```python
from build123d import *

# Parameters (mm, degrees)
F0_W     = 100
F0_H     = 40
F1_DEPTH = 3
F2_R     = 3
F3_W     = 18
F3_H     = 9
F4_DEPTH = 25
F5_R     = 4.49999
F6_R     = 4.49999


# Not quite as in the source:
# - a fillet or chamfer is up to 0.001 mm smaller than in the source, because OpenCascade refuses the exact size


with BuildPart() as f1:
    # F0 (on Top) → F1 (new body)
    with BuildSketch(Plane.XY):
        Rectangle(F0_W, F0_H)
    extrude(amount=F1_DEPTH)

    # F2
    f2_edges = [f1.edges().sort_by_distance(p)[0] for p in [
        (50, -20, 1.5),
        (50, 20, 1.5),
        (-50, -20, 1.5),
        (-50, 20, 1.5),
    ]]
    fillet(f2_edges, radius=F2_R)

    # F3 (on face) → F4 (cut)
    with BuildSketch(Plane.XY.offset(3)):
        with Locations((-35, 0)):
            Rectangle(F3_W, F3_H)
        with Locations((35, 0)):
            Rectangle(F3_W, F3_H)
    extrude(amount=-F4_DEPTH, mode=Mode.SUBTRACT)

    # F5 (radius 4.5 in the source; OpenCascade refuses exactly that, so slightly less here)
    f5_edges = [f1.edges().sort_by_distance(p)[0] for p in [
        (-44, 4.5, 1.5),
        (-26, 4.5, 1.5),
        (-26, -4.5, 1.5),
        (-44, -4.5, 1.5),
    ]]
    fillet(f5_edges, radius=F5_R)

    # F6 (radius 4.5 in the source; OpenCascade refuses exactly that, so slightly less here)
    f6_edges = [f1.edges().sort_by_distance(p)[0] for p in [
        (26, 4.5, 1.5),
        (44, 4.5, 1.5),
        (44, -4.5, 1.5),
        (26, -4.5, 1.5),
    ]]
    fillet(f6_edges, radius=F6_R)


solid = f1.part
```
The model under review builds one solid part; all positions refer to its coordinate system, in mm. A direction names the side the tool comes from. Give positions to 0.01 mm unless a question says otherwise; leave off trailing zeros.
(1) To check wall thickness, follow L1, parallel to Y at x = -30.5, z = 1.8; L2, parallel to X at y = -3, z = 0.8; L3, parallel to X at y = -1, z = 0.25. State the ranges of each line that lie inside material, in increasing order.
(2) For P1, Ø10, axis at x = 12, y = 2, coming from the -Z side, flat-tipped, find the tip position at first contact; note if it passes through.
(3) The part is to be moulded in two halves that separate along X. For faces 1 (the cylindrical face through (-49.14, 19.1, 1.52)), 2 (the flat face through (-35, 4.5, 2)), 3 (the cylindrical face through (42.647, -3.217, 1.479)), 4 (the flat face through (-1, 0, 3)), say which applies: released by +X, released by -X, zero draft, split by the parting line, or undercut.
(4) Tool access review of faces 5 (the cylindrical face through (-49.14, -19.1, 1.52)), 6 (the cylindrical face through (-42.647, 3.217, 1.479)): name each direction out of +Z, -Z, +X, -X, +Y, -Y from which nothing blocks a thin tool from reaching the whole face with its end or side.
(5) Consider section A-A, the plane z = 0.8. Give the number of separate pieces and of enclosed holes in the cut face, and give its area (3 significant figures).
Returned:
1. L1: y = -20 to -4.5, 4.5 to 20
1. L2: x = -50 to -42.85, -27.15 to 27.15, 42.85 to 50
1. L3: x = -50 to -43.89, -26.11 to 26.11, 43.89 to 50
2. P1: stops at z = 0
3. face 1: released by -X
3. face 2: undercut
3. face 3: undercut
3. face 4: zero draft
4. face 5: +Z, -Z, -X, -Y
4. face 6: +Z, -Z
5. separate pieces: 1
5. enclosed holes: 2
5. area: 3,700 mm2
